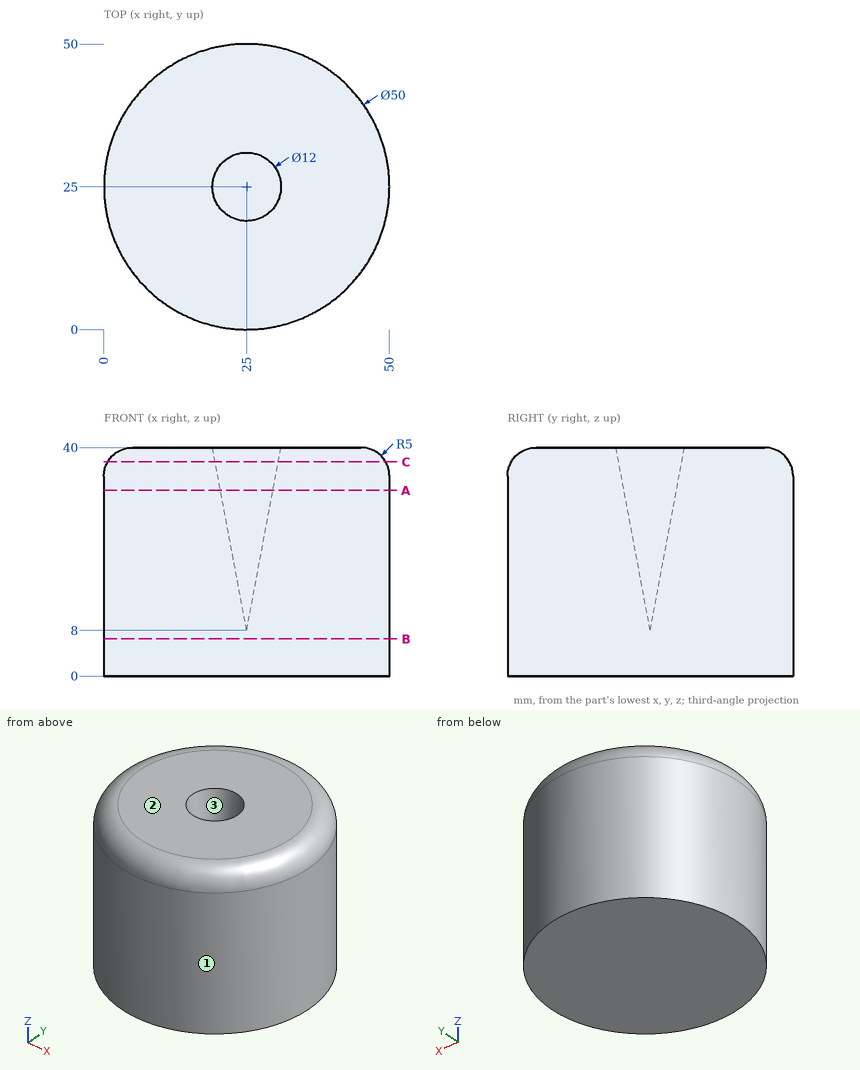
Design review of the part shown in the three views and the two pictorial views. Dimensions are in mm from the part's minimum x, y and z. Round coordinates to 2 decimals unless told otherwise and drop trailing zeros. Loops run counter-clockwise (first coordinate to the right, second up) from the corner with the lowest first, then second, coordinate; pieces in that order, holes last. Notation, with made-up numbers: (53, 32.25) - (93, 32.25) arc R19 cw to (93, 49.25) - close; hole circle Ø5 at (24, 39). An arc over 180 degrees is marked (long way). Use one line per item in the form item = value.
1) We need section C-C on z = 37.5. Write out the cut boundary in (x, y), then the cut area to 3 significant figures.
Solutions:
outline = circle Ø48.66 at (25, 25); hole circle Ø11.06 at (25, 25)
area = 1,760 mm2
2) Wall thickness on probe 1 along Z at (x, y) = (48, 26.5); probe 2 along Y at (x, z) = (14, 9); probe 3 along Y at (x, z) = (8, 33.5): over which ranges is each line inside the solid? List them lowest first.
Solutions:
probe_1 = 0 to 38.96
probe_2 = 2.55 to 47.45
probe_3 = 6.67 to 43.33
3) We need section A-A on z = 32.5. Write out the cut boundary in (x, y), then the cut area to 3 significant figures.
Solutions:
outline = circle Ø50 at (25, 25); hole circle Ø9.19 at (25, 25)
area = 1,900 mm2
4) Clearance check with flat-ended pins moving along their axes: P1, Ø4, axis at x = 16.5, z = 4.5, coming from the -Y side; P2, Ø2, axis at x = 30.5, z = 28, coming from the +Y side; P3, Ø2, axis at x = 44.5, z = 10, coming from the +Y side. State where each tip first meets the part, or that it passes through.
Solutions:
P1 = 0.86
P2 = 49.59
P3 = 41.82
5) Mouldability with a two-part tool opening along X and no side actions: class the marked faces 1, 2 and 3 as pulls with the +X half, pulls with the -X half, needs draft (parallel to the pull), parting line crosses it, or undercut.
Solutions:
face_1 = parting line crosses it
face_2 = needs draft
face_3 = undercut
6) We need section B-B on z = 6.5. Write out the cut boundary in (x, y), then the cut area to 3 significant figures.
Solutions:
outline = circle Ø50 at (25, 25)
area = 1,960 mm2
